Check sheet for the modelled part. Datum: model origin and axes. Units: mm. A direction names the side the tool comes from. Give positions to 0.01 mm unless a question says otherwise; leave off trailing zeros. Order: outer loops, then holes, each group sorted by start corner. A loop starts at its lowest first (then second) coordinate and runs counter-clockwise, first axis right, second up. Notation, with made-up numbers: (33, 29) -> (51, 29) arc R12 cw to (51, 41) -> close; hole circle Ø4 at (17, 79.5). An arc over 180 degrees is marked (long way). One line per question, with ' | ' between items.
```python
from build123d import *

# Parameters (mm, degrees)
F1_DEPTH = 110
F3_DEPTH = 10
F4_W     = 5.7648873329
F4_H     = 5.8702230453
F6_W     = 22
F6_H     = 20


with BuildPart() as f1:
    # F0 (on Front) → F1 (new body)
    with BuildSketch(Plane.XZ):
        Polygon((0, -2105), (0, 0), (-600, 0), (-600, -77), (-260, -77), (-260, -2105), align=None)
    extrude(amount=-F1_DEPTH)

    # F2 (on face) → F3 (join)
    with BuildSketch(Plane.XZ):
        Polygon((-239, -56), (-600, -56), (-600, -77), (-260, -77), (-260, -2105), (-239, -2105), align=None)
    extrude(amount=F3_DEPTH)

    # F5: sweep along a path in F5_path
    with BuildLine(Plane(origin=(-600, 110, -77), x_dir=(0, 0, 1), z_dir=(0, -1, 0))) as f5_path:
        Line((0, 0), (0, -340))
        Line((0, -340), (-2028, -340))
    # F4 (on face) → F5 (sweep)
    with BuildSketch(Plane(origin=(-600, 0, 0), x_dir=(0, -1, 0), z_dir=(-1, 0, 0))):
        with Locations((-107.1175563335, -74.0648884773)):
            Rectangle(F4_W, F4_H)
        Polygon((-104.2351126671, -77), (-110, -77), (-110, -85), (-33, -85), (-33, -77), align=None)
        Polygon((-130, -77), (-110, -77), (-110, -71.1297769547), (-110, 0), (-110, 2), (-130, 2), align=None)
    sweep(path=f5_path.line, transition=Transition.RIGHT)

    # F7: sweep along a path in F7_path
    with BuildLine(Plane(origin=(0, 110, 0), x_dir=(0, 0, 1), z_dir=(0, -1, 0))) as f7_path:
        Line((0, 0), (-2105, 0))
    # F6 (on face) → F7 (sweep)
    with BuildSketch(Plane.XY.offset(2)):
        with Locations((-11, 120)):
            Rectangle(F6_W, F6_H)
    sweep(path=f7_path.line)


solid = f1.part
```
Q1. Section check C-C (y = 81.5). Enter the section's corners in (x, z).
Result sheet:
outline: (-600, -85) -> (-268, -85) -> (-268, -2105) -> (0, -2105) -> (0, 0) -> (-600, 0) -> close
Q2. Depth check by flat-ended pin: pin 1 Ø1.5 at (x, y) = (-410, 109.5) entering from -Z; pin 2 Ø1 at (y, z) = (107.5, -1659) entering from +X; pin 3 Ø5 at (x, y) = (-244, 23.5) entering from +Z; pin 4 Ø10 at (x, y) = (-351.5, 123) entering from -Z. Enter the tip coordinate at first touch or a pass-through.
Result sheet:
pin 1: stops at z = -85 | pin 2: stops at x = 0 | pin 3: stops at z = 0 | pin 4: stops at z = -77
Q3. Section check B-B (x = -370.5). Enter the section's corners in (y, z).
Result sheet:
outline: (-10, -77) -> (33, -77) -> (33, -85) -> (110, -85) -> (110, -77) -> (130, -77) -> (130, 2) -> (110, 2) -> (110, 0) -> (0, 0) -> (0, -56) -> (-10, -56) -> close
Q4. Section check A-A (z = -1091.5). Enter the section's corners in (x, y).
Result sheet:
outline: (-268, 33) -> (-260, 33) -> (-260, -10) -> (-239, -10) -> (-239, 0) -> (0, 0) -> (0, 130) -> (-22, 130) -> (-22, 110) -> (-181, 110) -> (-181, 130) -> (-260, 130) -> (-260, 110) -> (-268, 110) -> close
Q5. Thickness scan on line 1 (X direction, y = 116, z = -1248.5); line 2 (Z direction, x = -72, y = 8); line 3 (Y direction, x = -72, z = -524.5). Record the ranges inside material, lowest first.
Result sheet:
line 1: x = -260 to -181, -22 to 0 | line 2: z = -2105 to 0 | line 3: y = 0 to 110
Q6. Access from +Z, -Z, +X, -X, +Y, -Y to the whole of each face (thin tool, end or side, straight path). Record for faces 1 (the face through (-268, 72, -1109)), 2 (the face through (-296, 54, 0)), 3 (the face through (-266, 33, -1096)), 4 (the face through (0, 64, -1066)), 5 (the face through (-600, 59, -41)).
Result sheet:
face 1: -Z, -X, +Y, -Y | face 2: +Z, +X, -X, -Y | face 3: -Z, -X, -Y | face 4: +Z, -Z, +X, +Y, -Y | face 5: +Z, -Z, -X, +Y, -Y
Q7. Section check D-D (x = -60). Enter the section's corners in (y, z), and give its area (3 significant figures).
Result sheet:
outline: (0, -2105) -> (110, -2105) -> (110, 0) -> (0, 0) -> close | area: 232,000 mm2
